Model file for the job. Use its own axes, mm. Coordinates: 2 decimals unless noted, no trailing zeros. Write each loop counter-clockwise with the first axis right and the second up, starting at its lowest first coordinate (ties: lowest second). Pieces come first, ordered by that corner, then holes. Notation, with made-up numbers: (14.25, -3) -> (64.25, -3) arc R13 ccw to (64.25, 17) -> close; hole circle Ø11 at (63, 24). An arc over 180 degrees is marked (long way). Answer as a JSON object with one key per item and string values. Group by question number.
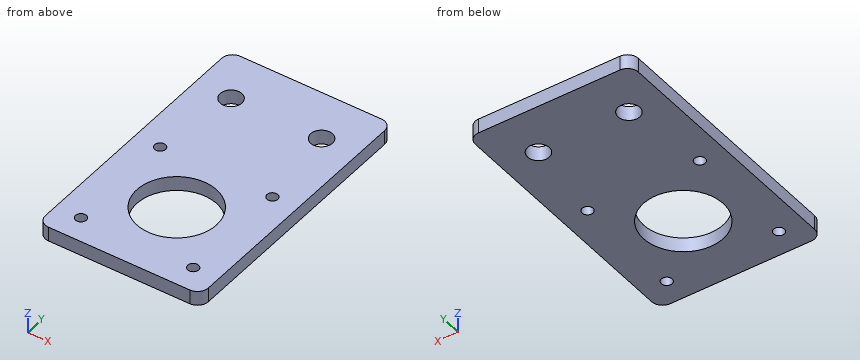
Autodesk Inventor part; units mm, degrees
ref_plane "YZ Plane" through (0, 0, 0) normal (1, 0, 0) x (0, 1, 0)
ref_plane "XZ Plane" through (0, 0, 0) normal (0, 1, 0) x (-1, 0, 0)
ref_plane "XY Plane" through (0, 0, 0) normal (0, 0, 1) x (1, 0, 0)
sketch "Szkic1" plane through (0, 0, 0) normal (0, 0, 1) x (1, 0, 0)
  line L0 (-9.5608, 1.5423) -> (35.4392, 1.5423)
  line L1 (35.4392, 1.5423) -> (35.4392, -73.4577)
  line L2 (26.8018, -148.3336) -> (-18.1982, -148.3336)
  line L3 (-9.5608, -73.4577) -> (-9.5608, 1.5423)
  line L4 (33.9392, -71.9577) -> (-8.0608, -71.9577)
  line L5 (-8.0608, -71.9577) -> (-8.0608, -29.9577)
  line L6 (-8.0608, -29.9577) -> (33.9392, -29.9577)
  line L7 (33.9392, -29.9577) -> (33.9392, -71.9577)
  line L8 (-9.5608, -73.4577) -> (35.4392, -73.4577)
  circle A0 centre (12.9392, -50.9577) radius 11
  circle A1 centre (-2.5608, -35.4577) radius 1.5
  circle A2 centre (28.4392, -35.4577) radius 1.5
  circle A3 centre (-2.5608, -66.4577) radius 1.5
  circle A4 centre (28.4392, -66.4577) radius 1.5
  circle A5 centre (0.4392, -11.9577) radius 3
  circle A6 centre (25.4392, -11.9577) radius 3
  point P0 (0, 0)
  dimension "d0" = 45
  dimension "d1" = 75
  dimension "d2" = 42
  dimension "d3" = 42
  dimension "d4" = 5.5
  dimension "d5" = 5.5
  dimension "d6" = 5.5
  dimension "d7" = 5.5
  dimension "d8" = 5.5
  dimension "d9" = 5.5
  dimension "d10" = 5.5
  dimension "d11" = 5.5
  dimension "d12" = 21
  dimension "d13" = 21
  dimension "d24" = 45
  dimension "d25" = 1.5
  dimension "d26" = 1.5
  dimension "d27" = 13.5
  dimension "d28" = 13.5
  dimension "d29" = 22
  dimension "d30" = 3
  dimension "d31" = 3
  dimension "d32" = 3
  dimension "d33" = 3
  dimension "d43" = 10
  dimension "d44" = 10
  dimension "d45" = 6
  dimension "d46" = 6
extrude "Wyciągnięcie proste2" add sketch "Szkic1" along normal blind 4 contours L0 L1 L8 L3 | L4 L5 L6 L7
fillet "Zaokrąglenie1" radius 3 4 edges at (35.4392, -73.4577, 2) (-9.5608, -73.4577, 2) (35.4392, 1.5423, 2) (-9.5608, 1.5423, 2)
equation "\"d25\" = -0.5 * d2 + 0.5 * d24"
properties part number "LC_ALU_4mm_Z_Axis_Stepper_Mount"
(1) Cut at C-C on z = 0.6. List the corners of the cut face in (x, y), plus the area to 3 significant figures.
(2) Pin check, flat tip, straight feed: pin 1 (5 mm diameter, centred on x = 8.5, y = -46, fed in from -Z). Stop position of the tip, or through.
(3) Cut at A-A on y = -61. List the corners of the cut face in (x, z), plus the area to 3 significant figures.
(4) Wall check: probe 1 along Y at (x, z) = (13.5, 0.25); probe 2 along Y at (x, z) = (-3, 1.8); probe 3 along X at (y, z) = (-14.5, 3.55). Give the ranges that are in metal, low to high.
(5) Cut at B-B on x = 10.5. List the corners of the cut face in (y, z), plus the area to 3 significant figures.
Results found:
{
 "1": {"outline": "(-9.56, -70.46) arc R3 ccw to (-6.56, -73.46) -> (32.44, -73.46) arc R3 ccw to (35.44, -70.46) -> (35.44, -1.46) arc R3 ccw to (32.44, 1.54) -> (-6.56, 1.54) arc R3 ccw to (-9.56, -1.46) -> close; hole circle Ø3 at (-2.56, -66.46); hole circle Ø3 at (-2.56, -35.46); hole circle Ø6 at (0.44, -11.96); hole circle Ø22 at (12.94, -50.96); hole circle Ø6 at (25.44, -11.96); hole circle Ø3 at (28.44, -66.46); hole circle Ø3 at (28.44, -35.46)", "area": "2,900 mm²"},
 "2": {"pin 1": "passes through"},
 "3": {"outline": "(-9.56, 0) -> (8.45, 0) -> (8.45, 4) -> (-9.56, 4) -> close; (17.43, 0) -> (35.44, 0) -> (35.44, 4) -> (17.43, 4) -> close", "area": "144 mm²"},
 "4": {"probe 1": "y = -73.46 to -61.94, -39.97 to 1.54", "probe 2": "y = -73.46 to -67.89, -65.02 to -36.89, -34.02 to 1.54", "probe 3": "x = -9.56 to -1.15, 2.03 to 23.85, 27.03 to 35.44"},
 "5": {"outline": "(-73.46, 0) -> (-61.68, 0) -> (-61.68, 4) -> (-73.46, 4) -> close; (-40.23, 0) -> (1.54, 0) -> (1.54, 4) -> (-40.23, 4) -> close", "area": "214 mm²"}
}
